```python
from build123d import *

# Parameters (mm, degrees)
SKETCH1_W            = 151.5
SKETCH1_H            = 151.5
BOSS_EXTRUDE1_DEPTH  = 2
SKETCH8_R            = 6
BOSS_EXTRUDE3_DEPTH  = 10
SKETCH9_R            = 5
CUT_EXTRUDE5_DEPTH   = 10
LPATTERN3_COUNT      = 2
LPATTERN3_PITCH      = 105
LPATTERN3_COUNT_DIR2 = 2
LPATTERN3_PITCH_DIR2 = 105
SKETCH10_W           = 10
SKETCH10_H           = 20
BOSS_EXTRUDE4_DEPTH  = 9
SKETCH11_W           = 11
SKETCH11_H           = 12
BOSS_EXTRUDE5_DEPTH  = 10
SKETCH13_W           = 10
SKETCH13_H           = 9
CUT_EXTRUDE6_DEPTH   = 10
SKETCH15_W           = 8
SKETCH15_H           = 15
CUT_EXTRUDE7_DEPTH   = 2


with BuildPart() as part:
    # Sketch1 → Boss-Extrude1 (new body)
    with BuildSketch(Plane(origin=(0, 0, 0), x_dir=(1, 0, 0), z_dir=(0, 1, 0))):
        with Locations((75.75, 75.75)):
            Rectangle(SKETCH1_W, SKETCH1_H)
    extrude(amount=BOSS_EXTRUDE1_DEPTH)

    # Sketch8 → Boss-Extrude3 (add)
    with BuildSketch(Plane(origin=(0, 0, 0), x_dir=(-1, 0, 0), z_dir=(0, -1, 0))):
        with Locations((-13, 13)):
            Circle(SKETCH8_R)
    boss_extrude3 = extrude(amount=BOSS_EXTRUDE3_DEPTH)

    # Sketch9 → Cut-Extrude5 (cut)
    with BuildSketch(Plane(origin=(0, 0, 0), x_dir=(1, 0, 0), z_dir=(0, 1, 0))):
        with Locations((13, 13)):
            Circle(SKETCH9_R)
    cut_extrude5 = extrude(amount=-CUT_EXTRUDE5_DEPTH, mode=Mode.SUBTRACT)

    # LPattern3: Boss-Extrude3, Cut-Extrude5 2 × 2
    with Locations(*[(i * LPATTERN3_PITCH, 0, -j * LPATTERN3_PITCH_DIR2) for i in range(LPATTERN3_COUNT) for j in range(LPATTERN3_COUNT_DIR2) if (i, j) != (0, 0)]):
        add(boss_extrude3)
        add(cut_extrude5, mode=Mode.SUBTRACT)

    # Sketch10 → Boss-Extrude4 (add)
    with BuildSketch(Plane(origin=(0, 0, 0), x_dir=(1, 0, 0), z_dir=(0, 1, 0))):
        with Locations((13, 151.5)):
            Rectangle(SKETCH10_W, SKETCH10_H)
    extrude(amount=-BOSS_EXTRUDE4_DEPTH)

    # Sketch11 → Boss-Extrude5 (add)
    with BuildSketch(Plane(origin=(0, 0, 0), x_dir=(-1, 0, 0), z_dir=(0, -1, 0))):
        with Locations((-146, 13)):
            Rectangle(SKETCH11_W, SKETCH11_H)
    extrude(amount=BOSS_EXTRUDE5_DEPTH)

    # Sketch13 → Cut-Extrude6 (cut)
    with BuildSketch(Plane(origin=(151.5, 0, 0), x_dir=(0, 0, -1), z_dir=(1, 0, 0))):
        with Locations((13, -4.5)):
            Rectangle(SKETCH13_W, SKETCH13_H)
    extrude(amount=-CUT_EXTRUDE6_DEPTH, mode=Mode.SUBTRACT)

    # Sketch15 → Cut-Extrude7 (cut)
    with BuildSketch(Plane(origin=(0, 0, 0), x_dir=(1, 0, 0), z_dir=(0, 1, 0))):
        with Locations((13, 34.25)):
            Rectangle(SKETCH15_W, SKETCH15_H)
    extrude(amount=CUT_EXTRUDE7_DEPTH, mode=Mode.SUBTRACT)


solid = part.part
```
Source: CAD feature listing. Evaluate the final solid. Frame: model axes, mm. A direction names the side the tool comes from. Coordinates: 2 decimals unless noted, no trailing zeros. Loops run counter-clockwise (first coordinate to the right, second up) from the corner with the lowest first, then second, coordinate; pieces in that order, holes last. Notation, with made-up numbers: M -4.75,-38.75 L 48.25,-38.75 A27 ccw 48.25,-8.75 Z; hole C 38.5,47 d10. An arc over 180 degrees is marked long. Use a Markdown table: item, result. Add a question column.
Q1. Material intervals for L1, parallel to Z at x = 13, y = -7; L2, parallel to X at y = -2.75, z = -118; L3, parallel to X at y = -3.5, z = -13, sorted ascending.
Q2. Section query A-A, the plane y = -6. State how many separate pieces and enclosed holes the cut face has, and give its area (3 significant figures).
Q3. Access query for faces 1 (the flat face through (13, -9, -152)), 2 (the flat face through (147, -5, -8)), 3 (the cylindrical face through (124, -5, -13)). Directions: +Z, -Z, +X, -X, +Y, -Y. A direction counts if a zero-diameter tool reaches every point of the face in a straight line with its end or side. Return the directions, or none.
Q4. Section query B-B, the plane x = 13. Return loops of the section in (y, z), and give its area (3 significant figures).
Q5. Section query C-C, the plane z = -13. Return loops of the section in (x, y), and give its area (3 significant figures).
Q6. Draft query along Z for faces 4 (the flat face through (146, -5, -7)), 5 (the flat face through (13, 0, -157)), 6 (the cylindrical face through (122.619, -4.93, -11.085)). Return one class per face: pulls with the +Z half, pulls with the -Z half, needs draft (parallel to the pull), parting line crosses it, or undercut.
Q7. Section query D-D, the plane x = 118. Return loops of the section in (y, z), and give its area (3 significant figures).
Q8. First-contact query: pin 1 (3 mm diameter, centred on x = 15, z = -119, fed in from -Y); pin 2 (2.5 mm diameter, centred on y = -4, z = -15.5, fed in from +X); pin 3 (2.5 mm diameter, centred on x = 146.5, y = -4, fed in from +Z). Flat tips, straight axial feed; report the tip coordinate or a pass-through.
Result:
| question | item | result |
|---|---|---|
| 1 | L1 | z = -161.5 to -141.5, -124 to -123, -113 to -112, -19 to -18, -8 to -7 |
| 1 | L2 | x = 7 to 8, 18 to 19, 112 to 113, 123 to 124 |
| 1 | L3 | x = 7 to 8, 18 to 19, 112 to 113, 123 to 124, 140.5 to 141.5 |
| 2 | separate pieces | 6 |
| 2 | enclosed holes | 4 |
| 2 | area | 370 mm2 |
| 3 | face 1 | -Z, +X, -X, -Y |
| 3 | face 2 | +X |
| 3 | face 3 | -Y |
| 4 | outline | M -10,-124 L 0,-124 L 0,-141.5 L -9,-141.5 L -9,-161.5 L 0,-161.5 L 0,-151.5 L 2,-151.5 L 2,-41.75 L 0,-41.75 L 0,-112 L -10,-112 L -10,-113 L 0,-113 L 0,-123 L -10,-123 Z; M -10,-19 L 0,-19 L 0,-26.75 L 2,-26.75 L 2,0 L 0,0 L 0,-7 L -10,-7 L -10,-8 L 0,-8 L 0,-18 L -10,-18 Z |
| 4 | area | 493 mm2 |
| 5 | outline | M 0,0 L 7,0 L 7,-10 L 8,-10 L 8,0 L 18,0 L 18,-10 L 19,-10 L 19,0 L 112,0 L 112,-10 L 113,-10 L 113,0 L 123,0 L 123,-10 L 124,-10 L 124,0 L 140.5,0 L 140.5,-10 L 151.5,-10 L 151.5,-9 L 141.5,-9 L 141.5,0 L 151.5,0 L 151.5,2 L 0,2 Z |
| 5 | area | 363 mm2 |
| 6 | face 4 | pulls with the +Z half |
| 6 | face 5 | needs draft |
| 6 | face 6 | undercut |
| 7 | outline | M -10,-124 L 0,-124 L 0,-151.5 L 2,-151.5 L 2,0 L 0,0 L 0,-7 L -10,-7 L -10,-8 L 0,-8 L 0,-18 L -10,-18 L -10,-19 L 0,-19 L 0,-112 L -10,-112 L -10,-113 L 0,-113 L 0,-123 L -10,-123 Z |
| 7 | area | 343 mm2 |
| 8 | pin 1 | stops at y = 0 |
| 8 | pin 2 | stops at x = 141.5 |
| 8 | pin 3 | stops at z = -7 |
